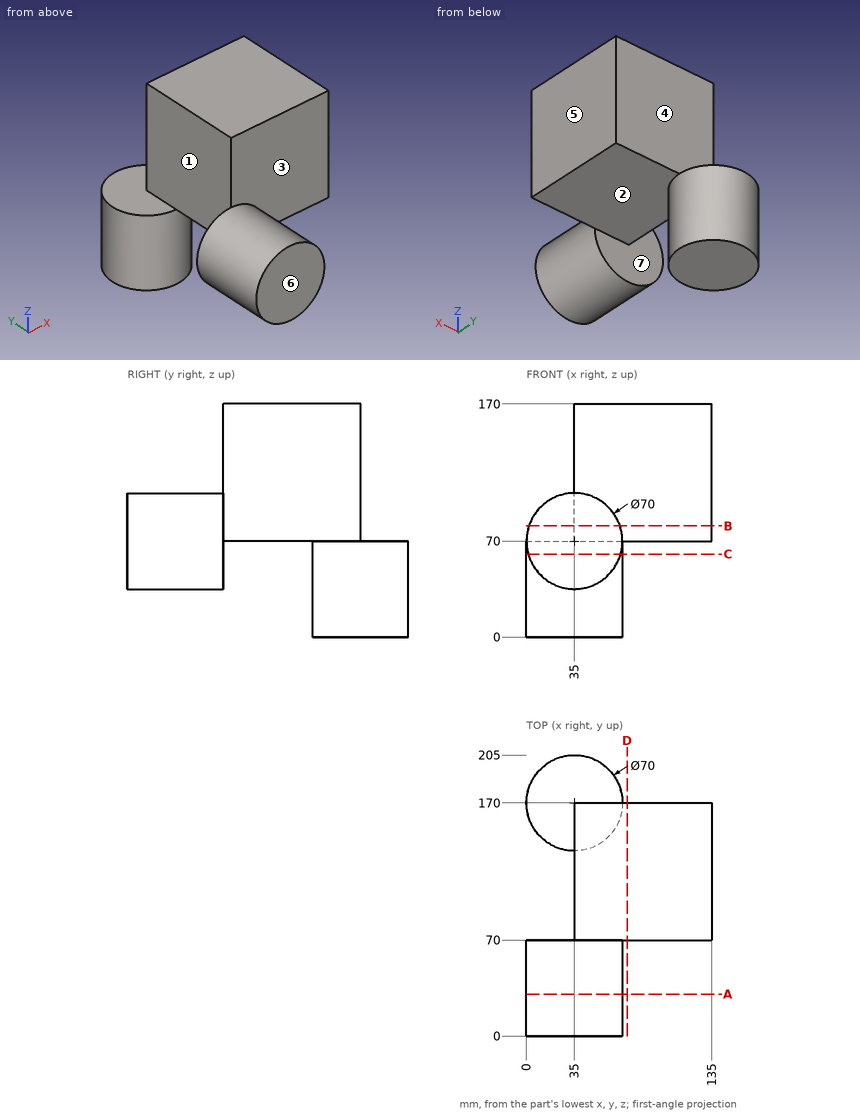
Verification items for this drawing (mm, ordinates from the low corner). A direction names the side the tool comes from. Coordinates: 2 decimals unless noted, no trailing zeros. Order: outer loops, then holes, each group sorted by start corner. A loop starts at its lowest first (then second) coordinate and runs counter-clockwise, first axis right, second up. Notation, with made-up numbers: (-34.75, 16.25) - (-4.75, 16.25) arc R10 cw to (-4.75, 31.25) - close; hole circle Ø7 at (80, 57). An arc over 180 degrees is marked (long way). Answer as a JSON object with one key per item and string values. Group by question number.
Item 1: Sectioned sample at A-A, the plane y = 30.5. Record the cut outline in (x, z), and give its area (3 significant figures).
Item 2: Sectioned sample at B-B, the plane z = 81. Record the cut outline in (x, y).
Item 3: Tool access check on the marked faces 1, 2, 3 and 4. Record the directions out of +Z, -Z, +X, -X, +Y, -Y that give a thin tool (end or side, any length) a straight path to the whole face; none if there is none.
Item 4: Draft check along Y on the marked faces 5, 6 and 7. Enter one of: +Y half, -Y half, draft (parallel to the pull), parting line (faces both ways), or undercut.
Item 5: Depth check by flat-ended pin: pin 1 Ø3 at (x, y) = (62.5, 62) entering from +Z; pin 2 Ø2 at (x, z) = (67, 45.5) entering from +Y; pin 3 Ø21 at (x, z) = (42.5, 55) entering from +Y. Enter the tip coordinate at first touch or a pass-through.
Item 6: Sectioned sample at C-C, the plane z = 60.5. Record the cut outline in (x, y).
Item 7: Sectioned sample at D-D, the plane x = 73.5. Record the cut outline in (y, z).
Item 8: Scan lines: probe 1 along Y at (x, z) = (99, 79); probe 2 along X at (y, z) = (159.5, 112.5); probe 3 along Z at (x, y) = (50.5, 177.5). Record each from-to range of solid material in increasing order.
Resolved:
{
 "1": {"outline": "circle Ø70 at (35, 70)", "area": "3,850 mm^2"},
 "2": {"outline": "(1.77, 0) - (68.23, 0) - (68.23, 70) - (135, 70) - (135, 170) - (35, 170) - (35, 70) - (1.77, 70) - close"},
 "3": {"face 1": "+Z, -X, +Y", "face 2": "-Z, +X", "face 3": "+Z, +X, -Y", "face 4": "+Z, +X, -X, +Y"},
 "4": {"face 5": "draft", "face 6": "-Y half", "face 7": "undercut"},
 "5": {"pin 1": "z = 93.43", "pin 2": "y = 186.25", "pin 3": "y = 205"},
 "6": {"outline": "circle Ø70 at (35, 170); (1.31, 0) - (68.69, 0) - (68.69, 70) - (1.31, 70) - close"},
 "7": {"outline": "(70, 70) - (170, 70) - (170, 170) - (70, 170) - close"},
 "8": {"probe 1": "70 to 170", "probe 2": "35 to 135", "probe 3": "0 to 70"}
}
